from build123d import *
from OCP.BRepFilletAPI import BRepFilletAPI_MakeChamfer

# Parameters (mm, degrees)
BOSS_EXTRUDE1_DEPTH            = 10
BOSS_EXTRUDE2_DEPTH            = 50
F_8_0MM_DOWEL_HOLE1_D          = 8
FILLET1_R                      = 2.5
CHAMFER1_SIZE                  = 1.5
CBORE_FOR_M5_SHCS1_D           = 5.5
CBORE_FOR_M5_SHCS1_CBORE_D     = 10
CBORE_FOR_M5_SHCS1_CBORE_DEPTH = 5
SKETCH9_R                      = 2.75
BOSS_EXTRUDE3_DEPTH            = 0.4
CHAMFER2_SIZE                  = 1
CHAMFER2_SIZE2                 = 1.732050808


with BuildPart() as part:
    # Sketch1 → Boss-Extrude1 (new, symmetric)
    with BuildSketch(Plane(origin=(0, 0, 0), x_dir=(1, 0, 0), z_dir=(0, 1, 0))):
        Polygon((12, 0), (-12, 0), (-12, -16), (-132.740728286, -16), (-12, 16.352380638), (12, 16.352380638), (132.740728286, -16), (12, -16), align=None)
    extrude(amount=BOSS_EXTRUDE1_DEPTH, both=True)

    # Sketch2 → Boss-Extrude2 (add, symmetric)
    with BuildSketch(Plane(origin=(0, 0, 0), x_dir=(1, 0, 0), z_dir=(0, 1, 0))):
        Polygon((-12, -16), (-12, 0), (12, 0), (12, -16), (22, -16), (22, 10), (-22, 10), (-22, -16), align=None)
    extrude(amount=BOSS_EXTRUDE2_DEPTH, both=True)

    # Ø8.0mm Dowel Hole1 (through all)
    with Locations(Plane(origin=(4.891942737, 0, -18.256978841), x_dir=(-0.96592582628907, 0, -0.2588190451025143), z_dir=(0.2588190451025143, 0, -0.96592582628907))):
        with Locations((-97.358802374, 0), (-67.358802374, 0), (-37.358802374, 0)):
            f_8_0mm_dowel_hole1 = Hole(F_8_0MM_DOWEL_HOLE1_D / 2)

    # Mirror1: Ø8.0mm Dowel Hole1 across plane
    add(f_8_0mm_dowel_hole1.mirror(Plane(origin=(0, 0, 0), x_dir=(0, 0, 1), z_dir=(1, 0, 0))), mode=Mode.SUBTRACT)

    # Fillet1
    fillet1_edges = [part.edges().sort_by_distance(p)[0] for p in [
        (-132.740728286, 0, 16),
        (-12, 0, -16.352380638),
        (12, 0, -16.352380638),
        (132.740728286, 0, 16),
        (-22, 30, 16),
        (22, 30, 16),
        (22, 30, -10),
        (-22, 30, -10),
        (-22, -30, 16),
        (22, -30, 16),
        (22, -30, -10),
        (-22, -30, -10),
    ]]
    fillet(fillet1_edges, radius=FILLET1_R)

    # Chamfer1
    chamfer1_edges = [part.edges().sort_by_distance(p)[0] for p in [
        (0, 10, -16.352380638),
        (-66.625671502, -10, 16),
        (-63.358153493, -10, -2.591004885),
        (63.358153493, -10, -2.591004885),
        (-116.229955158, -10, 13.826315481),
        (116.229955158, -10, 13.826315481),
        (-11.997184237, -10, -16.330992791),
        (11.997184237, -10, -16.330992791),
        (63.358153493, 10, -2.591004885),
        (-63.358153493, 10, -2.591004885),
        (-66.625671502, 10, 16),
        (-116.229955158, 10, 13.826315481),
        (116.229955158, 10, 13.826315481),
        (-11.997184237, 10, -16.330992791),
        (11.997184237, 10, -16.330992791),
        (-15.75, 50, 16),
        (-15.75, -50, 16),
        (-22, -50, 3),
        (0, -50, -10),
        (22, -50, 3),
        (-21.267766953, -50, -9.267766953),
        (21.267766953, -50, -9.267766953),
        (21.267766953, -50, 15.267766953),
        (-21.267766953, -50, 15.267766953),
        (-22, 50, 3),
        (22, 50, 3),
        (0, 50, -10),
        (-21.267766953, 50, -9.267766953),
        (21.267766953, 50, -9.267766953),
        (21.267766953, 50, 15.267766953),
        (-21.267766953, 50, 15.267766953),
        (-12, 0, 16),
        (12, 0, 16),
        (66.625671502, -10, 16),
        (66.625671502, 10, 16),
        (-12, -50, 8),
        (0, -50, 0),
        (12, -50, 8),
        (15.75, -50, 16),
        (-12, 50, 8),
        (0, 50, 0),
        (12, 50, 8),
        (15.75, 50, 16),
        (0, -10, -16.352380638),
    ]]
    chamfer(chamfer1_edges, length=CHAMFER1_SIZE)

    # CBORE for M5 SHCS1 (through all)
    with Locations(Plane(origin=(0, 0, -10), x_dir=(-1, 0, 0), z_dir=(0, 0, -1))):
        with Locations((0, 38), (0, -38)):
            CounterBoreHole(CBORE_FOR_M5_SHCS1_D / 2, CBORE_FOR_M5_SHCS1_CBORE_D / 2, CBORE_FOR_M5_SHCS1_CBORE_DEPTH)

    # Sketch9 → Boss-Extrude3 (add)
    with BuildSketch(Plane.XY):
        with Locations(Location((0, -38, 0), (0, 0, 180))):
            Circle(SKETCH9_R)
        with Locations(Location((0, 38, 0), (0, 0, 180))):
            Circle(SKETCH9_R)
    extrude(amount=-BOSS_EXTRUDE3_DEPTH)

    # Chamfer2: one chamfer whose edges measure the first distance from different faces: ONE call of the kernel's chamfer builder (chamfer() names one face for all edges)
    chamfer2_edges_1 = [part.edges().sort_by_distance(p)[0] for p in [
        (37.114071484, 0, -9.623085465),
        (66.091846273, 0, -1.858514112),
        (95.069621061, 0, 5.906057241),
    ]]
    chamfer2_side_1 = [part.faces().sort_by_distance(p)[0] for p in [
        (62.753662863, 0, -2.752977661),
    ]]
    chamfer2_edges_2 = [part.edges().sort_by_distance(p)[0] for p in [
        (-37.114071484, 0, -9.623085465),
        (-66.091846273, 0, -1.858514112),
        (-95.069621061, 0, 5.906057241),
    ]]
    chamfer2_side_2 = [part.faces().sort_by_distance(p)[0] for p in [
        (-62.753662863, 0, -2.752977661),
    ]]
    chamfer2 = BRepFilletAPI_MakeChamfer(part.part.solid().wrapped)
    for e in chamfer2_edges_1:
        chamfer2.Add(CHAMFER2_SIZE, CHAMFER2_SIZE2, e.wrapped, chamfer2_side_1[0].wrapped)  # the first distance lies on this face
    for e in chamfer2_edges_2:
        chamfer2.Add(CHAMFER2_SIZE, CHAMFER2_SIZE2, e.wrapped, chamfer2_side_2[0].wrapped)  # the first distance lies on this face
    add(Compound.cast(chamfer2.Shape()), mode=Mode.REPLACE)


solid = part.part
Can you work these out from the model? Positions are in its coordinate system, mm. A direction names the side the tool comes from. Coordinates: 2 decimals unless noted, no trailing zeros. Write each loop counter-clockwise with the first axis right and the second up, starting at its lowest first coordinate (ties: lowest second). Pieces come first, ordered by that corner, then holes. Notation, with made-up numbers: (8.25, 3.5) -> (35.25, 3.5) arc R27 cw to (35.25, 23.5) -> close; hole circle Ø1 at (-36.5, 31.25). An arc over 180 degrees is marked (long way). Answer as CSV lines item,"result".
1) Will these pins go through, and if not, where does the flat tip stop? P1, Ø4, axis at y = -26.5, z = 10, coming from the -X side; P2, Ø11.5, axis at x = -5, y = -24.5, coming from the -Z side; P3, Ø4, axis at x = -9, z = -13, coming from the +Y side; P4, Ø5, axis at x = -50.5, z = -10, coming from the -Y side.
Check result:
P1,"x = -22"
P2,"z = -10"
P3,"y = 10"
P4,"through"
2) On a 3-axis mill with a long thin cutter (end or side, diameter ignored), from which of +Z, -Z, +X, -X, +Y, -Y can I reach the whole of each face in a straight line? I mean faces 1 (the flat face through (0, -29, -10)), 2 (the flat face through (-64.07, 0.12, -2.4)), 3 (the cylindrical face through (-0.358, 40.727, -2.668)), 4 (the flat face through (63.881, -9.239, -1.685)), 5 (the flat face through (22, -29, 3)). Say none if no direction works.
Check result:
face 1,"-Z, +X, -X, -Y"
face 2,"-Z, -X, +Y, -Y"
face 3,"-Z"
face 4,"-Z, +X, -Y"
face 5,"+Z, -Z, +X, -Y"
3) If we section it at D-D on x = -88: Please give me the cut outline in (y, z).
Check result:
outline,"(-10, 5.56) -> (-8.5, 4.01) -> (8.5, 4.01) -> (10, 5.56) -> (10, 14.5) -> (8.5, 16) -> (-8.5, 16) -> (-10, 14.5) -> close"
4) If I drill on line 1 (Y direction, x = 0, z = -1.9); line 2 (Y direction, x = 0, z = -6); line 3 (X direction, y = 40, z = 6.5), over which ranges is the centre line in solid material (lowest first)? Write a range as from..to.
Check result:
line 1,"-50..-40.75, -35.25..35.25, 40.75..50"
line 2,"-50..-43, -33..33, 43..50"
line 3,"-22..-12, 12..22"
5) If we mould it in two halves opening along X, with no side actions, what happens to faces 6 (the flat face through (0, 30, -10)), 7 (the flat face through (-12, 1, 7)), 8 (the flat face through (-22, 30, 3)), 9 (the cylindrical face through (33.403, 0.176, 4.243))? For each: +X half, -X half, draft (parallel to the pull), parting line (faces both ways), or undercut.
Check result:
face 6,"draft"
face 7,"undercut"
face 8,"-X half"
face 9,"undercut"
6) If we section it at C-C on y = 15: Please give me the cut outline in (x, z), then the cut area to 3 significant figures.
Check result:
outline,"(-22, -7.5) arc R2.5 ccw to (-19.5, -10) -> (19.5, -10) arc R2.5 ccw to (22, -7.5) -> (22, 13.5) arc R2.5 ccw to (19.5, 16) -> (13.5, 16) -> (12, 14.5) -> (12, 0) -> (-12, 0) -> (-12, 14.5) -> (-13.5, 16) -> (-19.5, 16) arc R2.5 ccw to (-22, 13.5) -> close"
area,"752 mm²"
7) If we section it at A-A on y = 38: Please give me the cut outline in (x, z), then the cut area to 3 significant figures.
Check result:
outline,"(-22, -7.5) arc R2.5 ccw to (-19.5, -10) -> (-5, -10) -> (-5, -5) -> (-2.75, -5) -> (-2.75, -0.4) -> (2.75, -0.4) -> (2.75, -5) -> (5, -5) -> (5, -10) -> (19.5, -10) arc R2.5 ccw to (22, -7.5) -> (22, 13.5) arc R2.5 ccw to (19.5, 16) -> (13.5, 16) -> (12, 14.5) -> (12, 0) -> (-12, 0) -> (-12, 14.5) -> (-13.5, 16) -> (-19.5, 16) arc R2.5 ccw to (-22, 13.5) -> close"
area,"677 mm²"
